Could you check a few things on this model? Use its own coordinates, in mm. Face numbers are marked on the shaded views. Give positions to 0.01 mm unless a question says otherwise; leave off trailing zeros. Write each loop counter-clockwise with the first axis right and the second up, starting at its lowest first coordinate (ties: lowest second). Pieces come first, ordered by that corner, then holes. Notation, with made-up numbers: M 38.5,80.25 L 73.5,80.25 A16 cw 73.5,91.25 Z; hole C 32,24 d6. An arc over 180 degrees is marked long. Use one line per item in the form item = value.
from build123d import *

# Parameters (mm, degrees)
F0_W     = 100
F0_H     = 3
F2_W     = 12
F2_H     = 5
F3_DEPTH = 43.855205
F4_R     = 2.75
F5_DEPTH = 50


with BuildPart() as f1:
    # F0 (on Front) → F1 (revolve)
    with BuildSketch(Plane.XZ):
        with Locations((50, 13.05)):
            Rectangle(F0_W, F0_H)
    revolve(axis=Axis((1.032291, 0, 0), (1, 0, 0)))

    # F2 (on Right) → F3 (cut)
    with BuildSketch(Plane.YZ):
        with Locations((0, 15.755282)):
            Rectangle(F2_W, F2_H)
    extrude(amount=F3_DEPTH, mode=Mode.SUBTRACT)

    # F4 (on Right) → F5 (join)
    with BuildSketch(Plane.YZ):
        with Locations((0, -14.55)):
            Circle(F4_R)
    extrude(amount=F5_DEPTH)


solid = f1.part
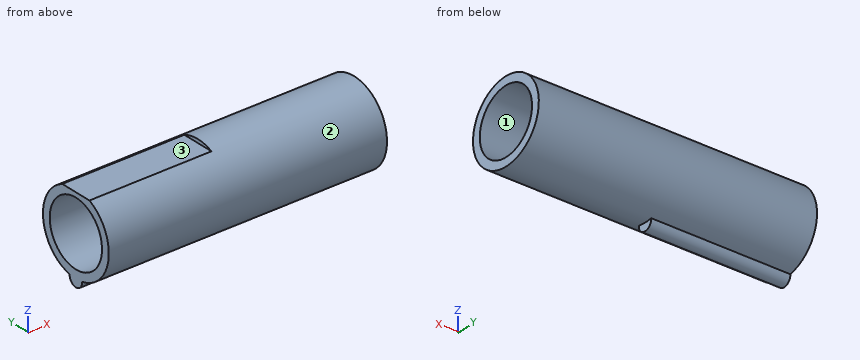
1) If I drill on L1, parallel to Y at x = 65, z = 0; L2, parallel to Z at x = 46, y = 0, over which ranges is the centre line in solid material (lowest first)?
Checked values:
L1 = -14.55 to -11.55, 11.55 to 14.55
L2 = -17.3 to -11.55, 11.55 to 14.55
2) I want a section at C-C, the plane x = 89. Please give me the cut outline in (y, z).
Checked values:
outline = C 0,0 d29.1; hole C 0,0 d23.1
3) I want a section at D-D, the plane z = -6. Please give me the cut outline in (x, y).
Checked values:
outline = M 0,-13.26 L 100,-13.26 L 100,-9.87 L 0,-9.87 Z; M 0,9.87 L 100,9.87 L 100,13.26 L 0,13.26 Z
4) I want a section at A-A, the plane z = 0. Please give me the cut outline in (x, y), plus the area to 3 significant figures.
Checked values:
outline = M 0,-14.55 L 100,-14.55 L 100,-11.55 L 0,-11.55 Z; M 0,11.55 L 100,11.55 L 100,14.55 L 0,14.55 Z
area = 600 mm2
5) I want a section at B-B, the plane y = 0. Please give me the cut outline in (x, z).
Checked values:
outline = M 0,-17.3 L 50,-17.3 L 50,-14.55 L 100,-14.55 L 100,-11.55 L 0,-11.55 Z; M 0,11.55 L 100,11.55 L 100,14.55 L 43.86,14.55 L 43.86,13.26 L 0,13.26 Z
6) For pin 1 Ø10 at (x, z) = (84.5, 10.5) entering from +Y; pin 2 Ø1.5 at (x, y) = (40, 1) entering from -Z; pin 3 Ø8 at (x, z) = (16, 10) entering from -Y, each with a flat end and sliding along its axis, tell me the tip position at first contact or that it passes through.
Checked values:
pin_1 = 13.47
pin_2 = -17.29
pin_3 = -13.26
7) Thinking about a two-plate mould opening in Z: for the marked faces 1, 2 and 3, which applies, released by +Z, released by -Z, zero draft, split by the parting line, or undercut?
Checked values:
face_1 = undercut
face_2 = split by the parting line
face_3 = released by +Z
